Read the model definition and answer for the solid it produces. Units are mm, in the model's axes. Give positions to 0.01 mm unless a question says otherwise; leave off trailing zeros. Write each loop counter-clockwise with the first axis right and the second up, starting at its lowest first coordinate (ties: lowest second). Pieces come first, ordered by that corner, then holes. Notation, with made-up numbers: M 32.25,10.5 L 61.25,10.5 A26 ccw 61.25,41.5 Z; hole C 33.25,-35 d2. An arc over 180 degrees is marked long. Use a Markdown table: item, result. Add a question column.
Item 1: A cutting plane is placed at A-A on x = 0. Determine the outline of the cut face in (y, z) (3 decimals).
Item 2: A cutting plane is placed at D-D on z = 80.5. Determine the outline of the cut face in (x, y) (3 decimals), then the cut area to 3 significant figures.
Item 3: The mould has two halves that part along Z. Classify faces 1 (the cylindrical face through (43.752, -0.027, 55.054)), 2 (the flat face through (43, -1.905, 43)): pulls with the +Z half, pulls with the -Z half, needs draft (parallel to the pull), parting line crosses it, or undercut.
Item 4: Given P1, Ø5.5, axis at x = -62.42, z = 43.71, coming from the +Y side; P2, Ø2, axis at x = 28, y = 0, coming from the +Z side; P3, Ø1, axis at y = 1, z = -21, coming from the +X side, each flat-ended and moving along its own axis, determine where each tip first touches the part or whether it passes through.
Item 5: A cutting plane is placed at B-B on x = -49.5. Determine the outline of the cut face in (y, z) (3 decimals), then the cut area to 3 significant figures.
Item 6: A cutting plane is placed at C-C on y = 0.6. Count the separate pieces of the cut face and the enclosed holes in it, then the cut area to 3 significant figures.
Item 7: Consider probe 1 along X at (y, z) = (1.4, -41); probe 2 along Z at (x, y) = (-60, -1.2); probe 3 along Z at (x, y) = (0, 1). Determine where each line is inside the solid, lowest interval first. Write a range as [from, to].
from build123d import *

# Parameters (mm, degrees)
F_98MM_6ID_CENTERING_RING_SKETCH_7_R = 53.34
CENTERING_RING_EXTRUDE_DEPTH         = 1.905
CENTERING_RING_EXTRUDE_DEPTH_BACK    = 1.905
CUT_EXTRUDE3_DEPTH                   = 4.81
CIRPATTERN1_COUNT                    = 6
CIRPATTERN1_ANGLE                    = 25
SKETCH5_R                            = 3.048
SKETCH5_R_2                          = 2.54
CUT_EXTRUDE4_DEPTH                   = 3.81


with BuildPart() as part:
    # 98mm - 6ID centering ring sketch_7 → Centering Ring Extrude (new body, two sides)
    with BuildSketch(Plane(origin=(0, 0, 0), x_dir=(1, 0, 0), z_dir=(0, 1, 0))) as centering_ring_extrude_sk:
        with BuildLine():
            Line((56.425744124, 3.175), (99.009105516, 3.175))
            ThreePointArc((99.009105516, 3.175), (70.045997744, 70.045997744), (3.175, 99.009105516))
            Line((3.175, 99.009105516), (3.175, 56.425744124))
            ThreePointArc((3.175, 56.425744124), (0, 56.515), (-3.175, 56.425744124))
            Line((-3.175, 56.425744124), (-3.175, 99.009105516))
            ThreePointArc((-3.175, 99.009105516), (-70.045997744, 70.045997744), (-99.009105516, 3.175))
            Line((-99.009105516, 3.175), (-56.425744124, 3.175))
            ThreePointArc((-56.425744124, 3.175), (-56.515, 0), (-56.425744124, -3.175))
            Line((-56.425744124, -3.175), (-99.009105516, -3.175))
            ThreePointArc((-99.009105516, -3.175), (-70.045997744, -70.045997744), (-3.175, -99.009105516))
            Line((-3.175, -99.009105516), (-3.175, -56.425744124))
            ThreePointArc((-3.175, -56.425744124), (0, -56.515), (3.175, -56.425744124))
            Line((3.175, -56.425744124), (3.175, -99.009105516))
            ThreePointArc((3.175, -99.009105516), (70.045997744, -70.045997744), (99.009105516, -3.175))
            Line((99.009105516, -3.175), (56.425744124, -3.175))
            ThreePointArc((56.425744124, -3.175), (56.515, 0), (56.425744124, 3.175))
        make_face()
        Circle(F_98MM_6ID_CENTERING_RING_SKETCH_7_R, mode=Mode.SUBTRACT)
        with BuildLine():
            ThreePointArc((99.06, 0), (99.047275562, 1.587703943), (99.009105516, 3.175))
            Line((99.009105516, 3.175), (56.425744124, 3.175))
            ThreePointArc((56.425744124, 3.175), (56.515, 0), (56.425744124, -3.175))
            Line((56.425744124, -3.175), (99.009105516, -3.175))
            ThreePointArc((99.009105516, -3.175), (99.047275562, -1.587703943), (99.06, 0))
        make_face()
        with BuildLine():
            Line((3.175, 56.425744124), (3.175, 99.009105516))
            ThreePointArc((3.175, 99.009105516), (0, 99.06), (-3.175, 99.009105516))
            Line((-3.175, 99.009105516), (-3.175, 56.425744124))
            ThreePointArc((-3.175, 56.425744124), (0, 56.515), (3.175, 56.425744124))
        make_face()
        with BuildLine():
            Line((-56.425744124, 3.175), (-99.009105516, 3.175))
            ThreePointArc((-99.009105516, 3.175), (-99.06, 0), (-99.009105516, -3.175))
            Line((-99.009105516, -3.175), (-56.425744124, -3.175))
            ThreePointArc((-56.425744124, -3.175), (-56.515, 0), (-56.425744124, 3.175))
        make_face()
        with BuildLine():
            ThreePointArc((-3.175, -99.009105516), (0, -99.06), (3.175, -99.009105516))
            Line((3.175, -99.009105516), (3.175, -56.425744124))
            ThreePointArc((3.175, -56.425744124), (0, -56.515), (-3.175, -56.425744124))
            Line((-3.175, -56.425744124), (-3.175, -99.009105516))
        make_face()
    extrude(amount=CENTERING_RING_EXTRUDE_DEPTH)
    extrude(centering_ring_extrude_sk.sketch, amount=-CENTERING_RING_EXTRUDE_DEPTH_BACK)

    # Sketch3 → Cut-Extrude3 (cut, through all)
    with BuildSketch(Plane(origin=(0, 1.905, 0), x_dir=(1, 0, 0), z_dir=(0, 1, 0))):
        with BuildLine():
            Line((-22.283651443, 96.521098618), (-19.141085214, 82.909148813))
            ThreePointArc((-19.141085214, 82.909148813), (-18.41684675, 83.073027246), (-17.691205772, 83.230579346))
            Line((-17.691205772, 83.230579346), (-20.595732092, 96.895301329))
            ThreePointArc((-20.595732092, 96.895301329), (-21.440508157, 96.711882465), (-22.283651443, 96.521098618))
        make_face()
    cut_extrude3 = extrude(amount=-CUT_EXTRUDE3_DEPTH, mode=Mode.SUBTRACT)

    # CirPattern1: Cut-Extrude3 ×6 about axis
    cirpattern1_axis = Axis((0, 0, 0), (0, -1, 0))
    for i in range(1, CIRPATTERN1_COUNT):
        add(cut_extrude3.rotate(cirpattern1_axis, i * CIRPATTERN1_ANGLE / (CIRPATTERN1_COUNT - 1)), mode=Mode.SUBTRACT)

    # Sketch5 → Cut-Extrude4 (cut)
    with BuildSketch(Plane.XZ.offset(1.905)):
        with Locations((-62.419385775, 43.70652445)):
            Circle(SKETCH5_R)
        with Locations((-44.082374272, 52.535327909)):
            Circle(SKETCH5_R_2)
        with Locations((44.082374272, 52.535327909)):
            Circle(SKETCH5_R_2)
        with Locations((62.419385775, 43.70652445)):
            Circle(SKETCH5_R)
        with Locations((62.419385775, -43.70652445)):
            Circle(SKETCH5_R)
        with Locations((44.082374272, -52.535327909)):
            Circle(SKETCH5_R_2)
        with Locations((-44.082374272, -52.535327909)):
            Circle(SKETCH5_R_2)
        with Locations((-62.419385775, -43.70652445)):
            Circle(SKETCH5_R)
    extrude(amount=-CUT_EXTRUDE4_DEPTH, mode=Mode.SUBTRACT)


solid = part.part
Filled in:
| question | item | result |
|---|---|---|
| 1 | outline | M -1.905,-99.06 L 1.905,-99.06 L 1.905,-53.34 L -1.905,-53.34 Z; M -1.905,53.34 L 1.905,53.34 L 1.905,99.06 L -1.905,99.06 Z |
| 2 | outline | M -57.729,-1.905 L 57.729,-1.905 L 57.729,1.905 L -57.729,1.905 Z |
| 2 | area | 440 mm² |
| 3 | face 1 | undercut |
| 3 | face 2 | needs draft |
| 4 | P1 | through |
| 4 | P2 | z = 95.31 |
| 4 | P3 | x = 96.92 |
| 5 | outline | M -1.905,-85.806 L 1.905,-85.806 L 1.905,-19.872 L -1.905,-19.872 Z; M -1.905,19.872 L 1.905,19.872 L 1.905,85.806 L -1.905,85.806 Z |
| 5 | area | 502 mm² |
| 6 | separate pieces | 1 |
| 6 | enclosed holes | 9 |
| 6 | area | 21,600 mm² |
| 7 | probe 1 | [-90.18, -63.82], [-61.02, -34.12], [34.12, 61.02], [63.82, 90.18] |
| 7 | probe 2 | [-78.82, -45.56], [-41.85, 41.85], [45.56, 78.82] |
| 7 | probe 3 | [-99.06, -53.34], [53.34, 99.06] |
